```python
from build123d import *

# Parameters (mm, degrees)
SKETCH1_W                = 80
SKETCH1_H                = 26.5
BOSS_EXTRUDE1_DEPTH      = 7
SKETCH5_W                = 80
SKETCH5_H                = 2.5
BOSS_EXTRUDE5_DEPTH      = 5
BOSS_EXTRUDE5_DEPTH_BACK = 31.5
SKETCH6_W                = 36.5
SKETCH6_H                = 2.5
BOSS_EXTRUDE6_DEPTH      = 20
BOSS_EXTRUDE6_DEPTH_BACK = 100
F_5_0MM_DOWEL_HOLE1_D    = 5


with BuildPart() as part:
    # Sketch1 → Boss-Extrude1 (new body)
    with BuildSketch(Plane(origin=(0, 0, 0), x_dir=(1, 0, 0), z_dir=(0, 1, 0))):
        with Locations((40, 13.25)):
            Rectangle(SKETCH1_W, SKETCH1_H)
    extrude(amount=BOSS_EXTRUDE1_DEPTH)

    # Sketch5 → Boss-Extrude5 (add, two sides)
    with BuildSketch(Plane.XY) as boss_extrude5_sk:
        with Locations((40, 1.25)):
            Rectangle(SKETCH5_W, SKETCH5_H)
    extrude(amount=BOSS_EXTRUDE5_DEPTH)
    extrude(boss_extrude5_sk.sketch, amount=-BOSS_EXTRUDE5_DEPTH_BACK)

    # Sketch6 → Boss-Extrude6 (add, two sides)
    with BuildSketch(Plane(origin=(80, 0, 0), x_dir=(0, 0, -1), z_dir=(1, 0, 0))) as boss_extrude6_sk:
        with Locations((13.25, 1.25)):
            Rectangle(SKETCH6_W, SKETCH6_H)
    extrude(amount=BOSS_EXTRUDE6_DEPTH)
    extrude(boss_extrude6_sk.sketch, amount=-BOSS_EXTRUDE6_DEPTH_BACK)

    # Ø5.0mm Dowel Hole1 (through all)
    with Locations(Plane(origin=(0, 2.5, 0), x_dir=(1, 0, 0), z_dir=(0, 1, 0))):
        with Locations((-10.375, 13.25), (90.375, 13.25)):
            Hole(F_5_0MM_DOWEL_HOLE1_D / 2)


solid = part.part
```
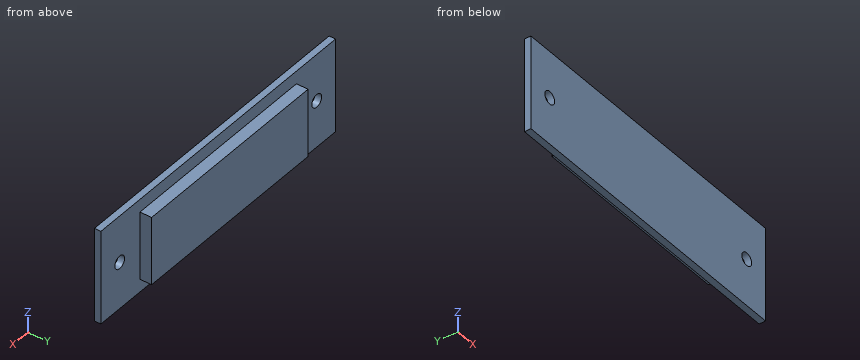
CAD build for the part. Positions are in the model's coordinates, mm. Round coordinates to 2 decimals unless told otherwise and drop trailing zeros. Order: outer loops, then holes, each group sorted by start corner. A loop starts at its lowest first (then second) coordinate and runs counter-clockwise, first axis right, second up. Notation, with made-up numbers: (38.5, 10) - (60.5, 10) arc R20 ccw to (60.5, 29) - close; hole circle Ø5 at (89, 2). An arc over 180 degrees is marked (long way). Answer as CSV lines item,"result". Start each with the question number.
1. Pin check, flat tips, straight feed: pin 1 (8 mm diameter, centred on x = -10.375, z = -13.25, fed in from +Y); pin 2 (1.3 mm diameter, centred on x = 30.5, y = 6, fed in from +Z); pin 3 (2 mm diameter, centred on y = 5, z = -14, fed in from -X); pin 4 (3 mm diameter, centred on x = 90.375, z = -13.25, fed in from +Y). Stop position of each tip, or through.
2. Saw through at D-D, the plane x = 36. Write the cut outline in (y, z), and give its area (4 significant figures).
3. Saw through at C-C, the plane z = -21. Write the cut outline in (x, y).
4. Saw through at B-B, the plane x = 91. Write the cut outline in (y, z).
5. Saw through at A-A, the plane z = -13.25. Write the cut outline in (x, y) (3 decimals), and give its area (3 significant figures).
6. Drill centre lines: L1, parallel to X at y = 1.6, z = -13.25 (3 decimals); L2, parallel to X at y = 5.5, z = -10; L3, parallel to Y at x = 74.5, z = 2. Where is each one in solid material? Low to high. Write a range as [from, to].
Model answer:
1,pin 1,"stops at y = 2.5"
1,pin 2,"stops at z = 0"
1,pin 3,"stops at x = 0"
1,pin 4,"passes through"
2,outline,"(0, -31.5) - (2.5, -31.5) - (2.5, -26.5) - (7, -26.5) - (7, 0) - (2.5, 0) - (2.5, 5) - (0, 5) - close"
2,area,"210.5 mm²"
3,outline,"(-20, 0) - (100, 0) - (100, 2.5) - (80, 2.5) - (80, 7) - (0, 7) - (0, 2.5) - (-20, 2.5) - close"
4,outline,"(0, -31.5) - (2.5, -31.5) - (2.5, -15.67) - (0, -15.67) - close; (0, -10.83) - (2.5, -10.83) - (2.5, 5) - (0, 5) - close"
5,outline,"(-20, 0) - (-12.875, 0) - (-12.875, 2.5) - (-20, 2.5) - close; (-7.875, 0) - (87.875, 0) - (87.875, 2.5) - (80, 2.5) - (80, 7) - (0, 7) - (0, 2.5) - (-7.875, 2.5) - close; (92.875, 0) - (100, 0) - (100, 2.5) - (92.875, 2.5) - close"
5,area,"635 mm²"
6,L1,"x = [-20, -12.875], [-7.875, 87.875], [92.875, 100]"
6,L2,"x = [0, 80]"
6,L3,"y = [0, 2.5]"
